from build123d import *

# Parameters (mm, degrees)
ESBO_O1_W                = 24
ESBO_O1_H                = 62
RESSALTO_EXTRUS_O1_DEPTH = 10
ESBO_O4_R                = 11
CORTE_EXTRUS_O1_DEPTH    = 1.5
CORTE_EXTRUS_O2_DEPTH    = 6
ESBO_O9_R                = 4.35
ESBO_O9_R_2              = 1.85
ESBO_O9_R_3              = 1.8
CORTE_EXTRUS_O4_DEPTH    = 11
ESBO_O11_OUTSIDE_W       = 25.446
ESBO_O11_OUTSIDE_H       = 77.446
CORTE_EXTRUS_O7_DEPTH    = 25


with BuildPart() as part:
    # Esboço1 → Ressalto-extrusão1 (new body)
    with BuildSketch(Plane.XY):
        Rectangle(ESBO_O1_W, ESBO_O1_H)
    extrude(amount=RESSALTO_EXTRUS_O1_DEPTH)

    # Esboço4 → Corte-extrusão1 (cut)
    with BuildSketch(Plane(origin=(0, 0, 10), x_dir=(-1, 0, 0), z_dir=(0, 0, -1))):
        Circle(ESBO_O4_R)
    extrude(amount=CORTE_EXTRUS_O1_DEPTH, mode=Mode.SUBTRACT)

    # Esboço6 → Corte-extrusão2 (cut)
    with BuildSketch(Plane.XY.offset(8.5)):
        Polygon((0, -7.909698688), (6.85, -3.954849344), (6.85, 3.954849344), (0, 7.909698688), (-6.85, 3.954849344), (-6.85, -3.954849344), align=None)
    extrude(amount=-CORTE_EXTRUS_O2_DEPTH, mode=Mode.SUBTRACT)

    # Esboço9 → Corte-extrusão4 (cut, through all)
    with BuildSketch(Plane.XY.offset(10)):
        Circle(ESBO_O9_R)
        with Locations((6, 26)):
            Circle(ESBO_O9_R_2)
        with Locations((-6, 26)):
            Circle(ESBO_O9_R_3)
        with Locations((-6, -26)):
            Circle(ESBO_O9_R_3)
        with Locations((6, -26)):
            Circle(ESBO_O9_R_3)
    extrude(amount=-CORTE_EXTRUS_O4_DEPTH, mode=Mode.SUBTRACT)

    # Esboço11 outside → Corte-extrusão7 (cut, through all)
    with BuildSketch(Plane.ZY.offset(12)):
        with Locations((5, 0)):
            Rectangle(ESBO_O11_OUTSIDE_W, ESBO_O11_OUTSIDE_H)
        Polygon((5.004562024, -21), (5, -31), (10, -31), (10, 31), (5, 31), (5.004562024, 21), (0, 15.995437976), (0, -15.995437976), align=None, mode=Mode.SUBTRACT)
    extrude(amount=-CORTE_EXTRUS_O7_DEPTH, mode=Mode.SUBTRACT)


solid = part.part
Input: part model. Units: mm. Frame: model coordinates. A direction names the side the tool comes from. Give positions to 0.01 mm unless a question says otherwise; leave off trailing zeros. Loops run counter-clockwise (first coordinate to the right, second up) from the corner with the lowest first, then second, coordinate; pieces in that order, holes last. Notation, with made-up numbers: M 57,12.25 L 94,12.25 A23 ccw 94,40.25 Z; hole C 3.5,40 d11. An arc over 180 degrees is marked long. Use one line per item in the form item = value.
1. First-contact query: pin 1 (3 mm diameter, centred on x = -6, y = 26, fed in from +Z); pin 2 (6.5 mm diameter, centred on x = 3, y = 5, fed in from +Z). Flat tips, straight axial feed; report the tip coordinate or a pass-through.
Numbers:
pin_1 = through
pin_2 = 8.5
2. Pull-direction query (Y, two-part tool) for faces 1 (the face through (0, 31, 7)), 2 (the face through (0, -31, 7)), 3 (the face through (5.759, 27.834, 7.536)); classes: released by +Y, released by -Y, zero draft, split by the parting line, or undercut.
Numbers:
face_1 = released by +Y
face_2 = released by -Y
face_3 = undercut
3. Section query C-C, the plane x = 6. Return the cut outline in (y, z), and give its area (3 significant figures).
Numbers:
outline = M -31,5 L -27.8,5 L -27.8,10 L -31,10 Z; M -24.2,5 L -21,5 L -16,0 L 16,0 L 21,5 L 24.15,5 L 24.15,10 L 9.22,10 L 9.22,8.5 L 4.45,8.5 L 4.45,2.5 L -4.45,2.5 L -4.45,8.5 L -9.22,8.5 L -9.22,10 L -24.2,10 Z; M 27.85,5 L 31,5 L 31,10 L 27.85,10 Z
area = 377 mm²
4. Section query A-A, the plane z = 7.5. Return the cut outline in (x, y), and give its area (3 significant figures).
Numbers:
outline = M -12,-31 L 12,-31 L 12,31 L -12,31 Z; hole C -6,-26 d3.6; hole C -6,26 d3.6; hole M -6.85,-3.95 L 0,-7.91 L 6.85,-3.95 L 6.85,3.95 L 0,7.91 L -6.85,3.95 Z; hole C 6,26 d3.7; hole C 6,-26 d3.6
area = 1,280 mm²
5. Section query B-B, the plane y = 0. Return the cut outline in (x, z).
Numbers:
outline = M -12,0 L -4.35,0 L -4.35,2.5 L -6.85,2.5 L -6.85,8.5 L -11,8.5 L -11,10 L -12,10 Z; M 4.35,0 L 12,0 L 12,10 L 11,10 L 11,8.5 L 6.85,8.5 L 6.85,2.5 L 4.35,2.5 Z
6. Line query: L1, parallel to X at y = 26, z = 8.15; L2, parallel to Y at x = 0.5, z = 9.75; L3, parallel to Y at x = -6, z = 6.9. Output: solid intervals per line, ascending.
Numbers:
L1 = -12 to -7.8, -4.2 to 4.15, 7.85 to 12
L2 = -31 to -10.99, 10.99 to 31
L3 = -31 to -27.8, -24.2 to -4.45, 4.45 to 24.2, 27.8 to 31
7. Reachability of faces 4 (the face through (-6.85, 0, 6)), 5 (the face through (6.968, -24.482, 7.536)) from +Z, -Z, +X, -X, +Y, -Y: full face, straight path, thin tool, end or side. Return the list, or none.
Numbers:
face_4 = +Z
face_5 = +Z, -Z
8. Section query D-D, the plane y = 26. Return the cut outline in (x, z).
Numbers:
outline = M -12,5 L -7.8,5 L -7.8,10 L -12,10 Z; M -4.2,5 L 4.15,5 L 4.15,10 L -4.2,10 Z; M 7.85,5 L 12,5 L 12,10 L 7.85,10 Z
